Design review of the part built by this model. Coordinates are the model's own, in mm. Face numbers are marked on the shaded views. A direction names the side the tool comes from. Coordinates: 2 decimals unless noted, no trailing zeros. Order: outer loops, then holes, each group sorted by start corner. A loop starts at its lowest first (then second) coordinate and runs counter-clockwise, first axis right, second up. Notation, with made-up numbers: (-12.5, 35.25) - (40.5, 35.25) arc R26 cw to (40.5, 56.25) - close; hole circle Ø2 at (46.25, 28.25). An arc over 180 degrees is marked (long way). Write item = value, one per line. Start each with the question number.
Autodesk Inventor part; units mm, degrees
ref_plane "YZ Plane" through (0, 0, 0) normal (1, 0, 0) x (0, 1, 0)
ref_plane "XZ Plane" through (0, 0, 0) normal (0, 1, 0) x (-1, 0, 0)
ref_plane "XY Plane" through (0, 0, 0) normal (0, 0, 1) x (1, 0, 0)
sketch "Sketch1" plane through (0, 0, 0) normal (0, 0, 1) x (1, 0, 0)
  line L0 (-35, 45) -> (35, 45)
  line L1 (35, 45) -> (35, -45)
  line L2 (35, -45) -> (-35, -45)
  line L3 (-35, -45) -> (-35, 45)
  point P0 (0, 0)
  point P1 (0, 45)
  point P2 (-35, 0)
  dimension "d0" = 70
  dimension "d1" = 90
extrude "Extrusion1" add sketch "Sketch1" along normal blind 45
sketch "Sketch2" plane through (0, 0, 45) normal (0, 0, 1) x (1, 0, 0)
  line L0 (-25.3, 42) -> (25.3, 42)
  line L1 (25.3, 42) -> (25.3, -35)
  line L2 (25.3, -35) -> (-25.3, -35)
  line L3 (-25.3, -35) -> (-25.3, 42)
  line L4 (-35, 45) -> (-35, -45)
  line L5 (35, -45) -> (35, 45)
  line L6 (-35, -45) -> (35, -45)
  line L7 (35, 45) -> (-35, 45)
  point P0 (0, 0)
  dimension "d4" = 9.7
  dimension "d5" = 9.7
  dimension "d6" = 10
  dimension "d7" = 3
extrude "Extrusion2" cut sketch "Sketch2" against normal blind 42 contours L0 L1 L2 L3
sketch "Sketch3" plane through (-35, 45, 0) normal (0, 1, 0) x (1, 0, 0)
  line L0 (60.3, -45) -> (9.7, -45)
  line L1 (9.7, -45) -> (9.7, -41.5)
  line L2 (9.7, -41.5) -> (60.3, -41.5)
  line L3 (60.3, -41.5) -> (60.3, -45)
  line L4 (9.7, -45) -> (9.7, -3)
  line L5 (60.3, -45) -> (60.3, -3)
  line L6 (70, -45) -> (0, -45)
  point P0 (35, 0)
  dimension "d10" = 3.5
extrude "Extrusion3" cut sketch "Sketch3" against normal up to surface (3 mm away)
sketch "Sketch5" plane through (0, 0, 45) normal (0, 0, 1) x (1, 0, 0)
  line L0 (-33, 45) -> (-25, 45)
  line L1 (-25, 45) -> (25, 45)
  line L2 (25, 45) -> (33, 45)
  line L3 (33, 45) -> (35, 43)
  line L4 (35, 43) -> (35, -43)
  line L5 (35, -43) -> (33, -45)
  line L6 (33, -45) -> (-33, -45)
  line L7 (-33, -45) -> (-35, -43)
  line L8 (-35, -43) -> (-35, 43)
  line L9 (-35, 43) -> (-33, 45)
  line L10 (-25, -30) -> (-25, 45)
  line L11 (25, -30) -> (-25, -30)
  line L12 (25, 45) -> (25, -30)
  circle A0 centre (-30, 40) radius 2
  circle A1 centre (30, -25) radius 2
  circle A2 centre (-15, -40) radius 2
  circle A3 centre (15, -40) radius 2
  circle A4 centre (30, 40) radius 2
  circle A5 centre (-30, -25) radius 2
  line L13 (14.15, -21.6) -> (14.15, 28.85)
  arc A6 (14.15, 28.85) -> (11.65, 31.35) centre (11.65, 28.85) ccw
  line L14 (11.65, 31.35) -> (-12.5, 31.35)
  arc A7 (-12.5, 31.35) -> (-15, 28.85) centre (-12.5, 28.85) ccw
  line L15 (-15, 28.85) -> (-15, -21.6)
  arc A8 (-15, -21.6) -> (-12.5, -24.1) centre (-12.5, -21.6) ccw
  line L16 (-12.5, -24.1) -> (11.65, -24.1)
  arc A9 (11.65, -24.1) -> (14.15, -21.6) centre (11.65, -21.6) ccw
  circle A10 centre (20.135, 3.655) radius 2
  circle A11 centre (-19.865, 3.655) radius 2
  point P0 (0, 0)
hole "Hole2" at (-30, 40, 45) at (30, 40, 45) at (30, -25, 45) at (15, -40, 45) at (-15, -40, 45) at (-30, -25, 45) direction (0, 0, -1) diameter 2.459 depth 30 tip angle 118
sketch "Sketch6" plane through (-25.3, -35, 45) normal (0, 1, 0) x (1, 0, 0)
  line L0 (50.6, 0) -> (0, 0)
  line L1 (0, 0) -> (0, 42)
  line L2 (50.6, 0) -> (50.6, 42)
  point P0 (25.3, 45)
  point P1 (10, 10)
  point P2 (25.3, 10)
  point P3 (25.3, 0)
  dimension "d30" = 10
  dimension "d31" = 10
hole "Hole3" at (0, -35, 35) direction (0, -1, 0) diameter 6 end through all countersink diameter 12 countersink angle 90
sketch "Sketch8" plane through (35, -45, 0) normal (1, 0, 0) x (0, 0, -1)
  line L0 (-45, 10) -> (0, 10)
  line L1 (0, 10) -> (0, -40)
  line L2 (0, -40) -> (-45, -40)
  line L3 (-45, -40) -> (-45, 10)
  line L4 (0, 0) -> (-45, 0)
  line L5 (-45, 0) -> (-45, 90)
  line L6 (0, 0) -> (0, 90)
  circle A0 centre (-35, -10) radius 3.5
  circle A1 centre (-10, -10) radius 3.5
  circle A2 centre (-35, -30) radius 3.5
  circle A3 centre (-10, -30) radius 3.5
  point P0 (0, 45)
  dimension "d42" = 10
  dimension "d43" = 40
  dimension "d44" = 7
  dimension "d45" = 7
  dimension "d46" = 10
  dimension "d47" = 10
  dimension "d48" = 10
  dimension "d59" = 10
extrude "Extrusion4" add sketch "Sketch8" along normal blind 10
fillet "Fillet1" radius 10 2 edges at (35, -35, 22.5) (45, -35, 22.5)
chamfer "Chamfer2" distance 2 angle 45 3 edges at (35, 45, 22.5) (-35, 45, 22.5) (-35, -45, 22.5)
sketch "Sketch9" plane through (-25.3, -35, 45) normal (0, 1, 0) x (1, 0, 0)
  circle A0 centre (25.3, 33) radius 7.5
  line L0 (50.6, 42) -> (0, 42)
  point P0 (25.3, 45)
  point P1 (25.3, 42)
  dimension "d55" = 15
  dimension "d56" = 9
extrude "Extrusion5" cut sketch "Sketch9" against normal through all
sketch "Sketch10" plane through (0, 0, 45) normal (0, 0, 1) x (1, 0, 0)
  line L0 (-32, 35) -> (32, 35)
  line L1 (32, 35) -> (32, -20)
  line L2 (32, -20) -> (-32, -20)
  line L3 (-32, -20) -> (-32, 35)
  line L4 (-25.3, -35) -> (-25.3, 45)
  line L5 (-35, 43) -> (-35, -43)
  circle A0 centre (-30, 40) radius 1.2295
  circle A1 centre (-30, -25) radius 1.2295
  point P0 (0, 0)
  point P1 (0, 35)
  point P2 (-32, 7.5)
  dimension "d60" = 3
  dimension "d61" = 5
  dimension "d62" = 5
extrude "Extrusion6" cut sketch "Sketch10" against normal up to surface (42 mm away) contours L0 L4 L2 L3 | L0 L1 L2 L4
fillet "Fillet2" radius 3 11 edges at (-25.3, -20, 24) (-32, -20, 24) (-32, 35, 24) (-25.3, 35, 24) (25.3, 42, 22.25) (25.3, 35, 24) (32, 35, 24) (32, -20, 24) (25.3, -20, 24) (25.3, -35, 24) (-25.3, -35, 24)
equation "\"d5\" = d4"
properties part number "0008-10-051 Cutie Priza"
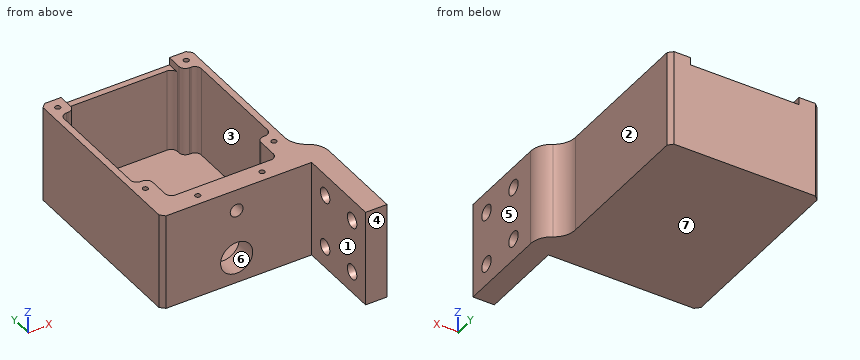
Item 1: Mouldability with a two-part tool opening along X and no side actions: class the marked faces 5, 6 and 7 as +X half, -X half, draft (parallel to the pull), parting line (faces both ways), or undercut.
Item 2: For P1, Ø2, axis at y = 42, z = 24.5, coming from the +X side; P2, Ø8, axis at x = 3.5, y = 20.5, coming from the +Z side; P3, Ø1.5, axis at x = -15.5, z = 10, coming from the -Y side; P4, Ø6.5, axis at y = -55, z = 10, coming from the +X side, all flat-tipped, find the tip position at first contact; note any pin that passes through.
Item 3: Add section C-C on x = 21. Give the boundary of the cut face in (y, z), plus the area to 4 significant figures.
Item 4: For line 1 (Z direction, x = 0, y = -40.5); line 2 (X direction, y = -25, z = 33.5); line 3 (Y direction, x = 15, z = 22), list the stretches that pass through material, from the lowest coordinate up.
Item 5: Add section B-B on y = 3. Give the boundary of the cut face in (x, z), plus the area to 3 significant figures.
Item 6: For the marked faces 1, 2, 3 and 4, list the 3-axis set-ups (+Z, -Z, +X, -X, +Y, -Y) from which the entire face can be reached by the end or side of a thin tool; tool diameter is ignored.
Item 7: Add section D-D on z = 21.5. State how many separate pieces and enclosed holes the cut face has, plus the area to 3 significant figures.
Item 8: Add section A-A on y = -55. Give the boundary of the cut face in (x, z), plus the area to 3 significant figures.
Worked out:
q1.face_5 = +X half
q1.face_6 = undercut
q1.face_7 = draft
q2.P1 = 35
q2.P2 = 3
q2.P3 = -45
q2.P4 = through
q3.outline = (-45, 0) - (45, 0) - (45, 41.5) - (42, 41.5) - (42, 3) - (-35, 3) - (-35, 45) - (-45, 45) - close
q3.area = 805.5 mm2
q4.line_1 = 0 to 4.5, 19.5 to 32, 38 to 45
q4.line_2 = -35 to -31.23, -28.77 to -25.3, 25.3 to 28.77, 31.23 to 35
q4.line_3 = -45 to -41.23, -38.77 to -35, 42 to 45
q5.outline = (-35, 0) - (35, 0) - (35, 45) - (32, 45) - (32, 3) - (-32, 3) - (-32, 45) - (-35, 45) - close
q5.area = 462 mm2
q6.face_1 = +Z, -Z, -X, -Y
q6.face_2 = +Z, -Z, +X, +Y
q6.face_3 = +Z
q6.face_4 = +Z, -Z, +X, -X, -Y
q7.separate_pieces = 1
q7.enclosed_holes = 7
q7.area = 2,150 mm2
q8.outline = (35, 0) - (45, 0) - (45, 6.5) - (35, 6.5) - close; (35, 13.5) - (45, 13.5) - (45, 31.5) - (35, 31.5) - close; (35, 38.5) - (45, 38.5) - (45, 45) - (35, 45) - close
q8.area = 310 mm2
